The figure shows three views and two pictorial views of one solid part (mm, origin at its lowest corner). Answer the questions. Coordinates: 2 decimals unless noted, no trailing zeros. Loops run counter-clockwise (first coordinate to the right, second up) from the corner with the lowest first, then second, coordinate; pieces in that order, holes last. Notation, with made-up numbers: (-0.75, 16.5) - (55.25, 16.5) arc R25 ccw to (55.25, 31.5) - close; hole circle Ø1 at (56.25, 61). An arc over 180 degrees is marked (long way). Return JSON: item names as keys, results as strings. Group by question number.
1. Section C-C (y = 1.3) is taken. State how many separate pieces and enclosed holes the cut face has.
2. Find the intervals of material crossed by line 1 along Y through (x, z) = (4.75, 47); line 2 along X through (y, z) = (1.05, 22) (1 decimal); line 3 along Z through (x, y) = (25.25, 0.85), in increasing order.
3. Each of these flat-tipped pins is pushed along its axis until it touches: P1, Ø0.8, axis at x = 6, y = 1, coming from the -Z side; P2, Ø4.5, axis at x = 14.29, z = 15.69, coming from the +Y side; P3, Ø4, axis at x = 25, z = 46.5, coming from the +Y side; P4, Ø0.5, axis at y = 1, z = 8.5, coming from the +X side. Where does it stop, or does it pass through?
4. Section B-B (z = 16) is taken. Write down the section's boundary in (x, y).
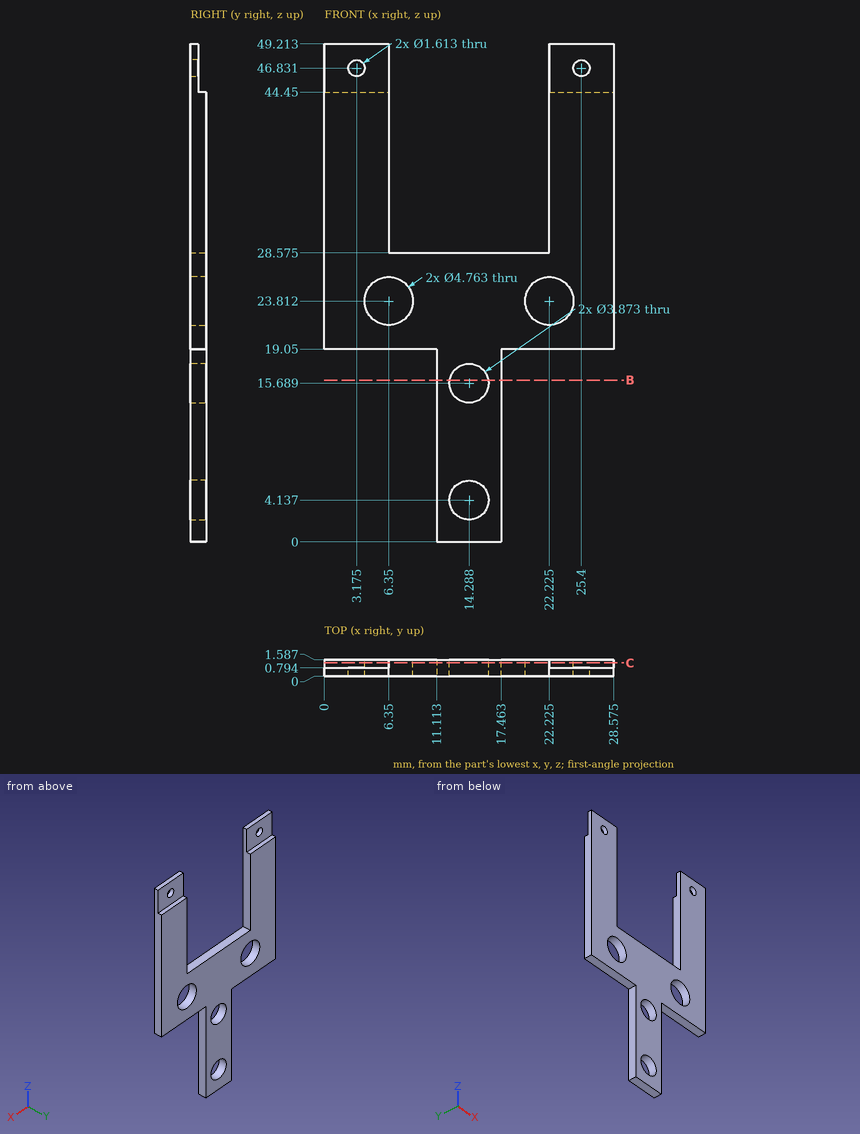
The answers:
{
 "1": {"separate pieces": "1", "enclosed holes": "4"},
 "2": {"line 1": "y = 0 to 0.79", "line 2": "x = 0 to 4.8, 7.9 to 20.7, 23.8 to 28.6", "line 3": "z = 19.05 to 44.45"},
 "3": {"P1": "stops at z = 19.05", "P2": "stops at y = 1.59", "P3": "stops at y = 0.79", "P4": "stops at x = 17.46"},
 "4": {"outline": "(11.11, 0) - (12.38, 0) - (12.38, 1.59) - (11.11, 1.59) - close; (16.2, 0) - (17.46, 0) - (17.46, 1.59) - (16.2, 1.59) - close"}
}
